Design review of the part built by this model. Coordinates are the model's own, in mm. Give positions to 0.01 mm unless a question says otherwise; leave off trailing zeros. Loops run counter-clockwise (first coordinate to the right, second up) from the corner with the lowest first, then second, coordinate; pieces in that order, holes last. Notation, with made-up numbers: (31.25, 7) -> (85.25, 7) arc R10 ccw to (85.25, 17) -> close; hole circle Ø10 at (88.5, 15). An arc over 180 degrees is marked (long way). Use CSV: the item, a comma, the result in double quotes. Start each with the question number.
Item 1: Wall thickness on line 1 along Y through (x, z) = (34, 2.8); line 2 along Y through (x, z) = (38.5, 3.25); line 3 along X through (y, z) = (18, 0.95): over which ranges is each line inside the solid? List them lowest first. Write a range as from..to.
Item 2: Clearance check with flat-ended pins moving along their axes: pin 1 (2 mm diameter, centred on y = 14.5, z = 1.5, fed in from -X); pin 2 (2 mm diameter, centred on x = 61.5, z = 1.5, fed in from +Y); pin 3 (1.5 mm diameter, centred on y = 76, z = 3, fed in from +X). State where each tip first meets the part, or that it passes through.
Item 3: We need section A-A (x = 91.5). State the section outline as (y, z) points.
Item 4: We need section B-B (y = 18). State the section outline as (x, z) points, plus the area to 3 significant figures.
from build123d import *

# Parameters (mm, degrees)
F0_W     = 100
F0_H     = 119
F1_DEPTH = 4
F2_W     = 4
F2_H     = 10
F2_W_2   = 8
F2_H_2   = 4
F3_DEPTH = 4.001
F5_DEPTH = 4


with BuildPart() as f1:
    # F0 (on Top) → F1 (new body)
    with BuildSketch(Plane.XY):
        with Locations((50, 59.5)):
            Rectangle(F0_W, F0_H)
    extrude(amount=F1_DEPTH)

    # F2 (on face) → F3 (cut, through all)
    with BuildSketch(Plane.XY.offset(4)):
        with Locations((98, 15)):
            Rectangle(F2_W, F2_H)
        with Locations((98, 35)):
            Rectangle(F2_W, F2_H)
        with Locations((98, 55)):
            Rectangle(F2_W, F2_H)
        with Locations((98, 75)):
            Rectangle(F2_W, F2_H)
        with Locations((98, 95)):
            Rectangle(F2_W, F2_H)
        with Locations((98, 115)):
            Rectangle(F2_W, F2_H)
        with Locations((2, 15)):
            Rectangle(F2_W, F2_H)
        with Locations((2, 35)):
            Rectangle(F2_W, F2_H)
        with Locations((2, 55)):
            Rectangle(F2_W, F2_H)
        with Locations((2, 75)):
            Rectangle(F2_W, F2_H)
        with Locations((2, 95)):
            Rectangle(F2_W, F2_H)
        with Locations((2, 115)):
            Rectangle(F2_W, F2_H)
        with Locations((16, 117)):
            Rectangle(F2_W_2, F2_H_2)
        with Locations((32, 117)):
            Rectangle(F2_W_2, F2_H_2)
        with Locations((84, 117)):
            Rectangle(F2_W_2, F2_H_2)
        with Locations((68, 117)):
            Rectangle(F2_W_2, F2_H_2)
    extrude(amount=-F3_DEPTH, mode=Mode.SUBTRACT)

    # F4 (on face) → F5 (join)
    with BuildSketch(Plane.XY.offset(4)):
        Polygon((42, 127), (40, 119), (60, 119), (58, 127), align=None)
    extrude(amount=-F5_DEPTH)


solid = f1.part
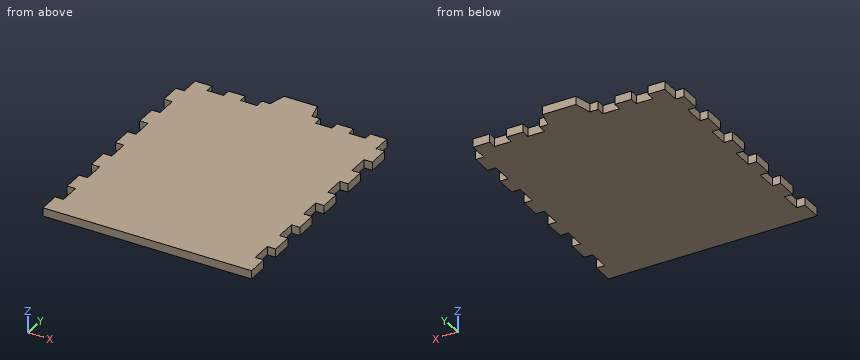
Results found:
1,line 1,"0..115"
1,line 2,"0..119"
1,line 3,"4..96"
2,pin 1,"x = 4"
2,pin 2,"y = 119"
2,pin 3,"x = 96"
3,outline,"(0, 0) -> (119, 0) -> (119, 4) -> (0, 4) -> close"
4,outline,"(4, 0) -> (96, 0) -> (96, 4) -> (4, 4) -> close"
4,area,"368 mm²"
